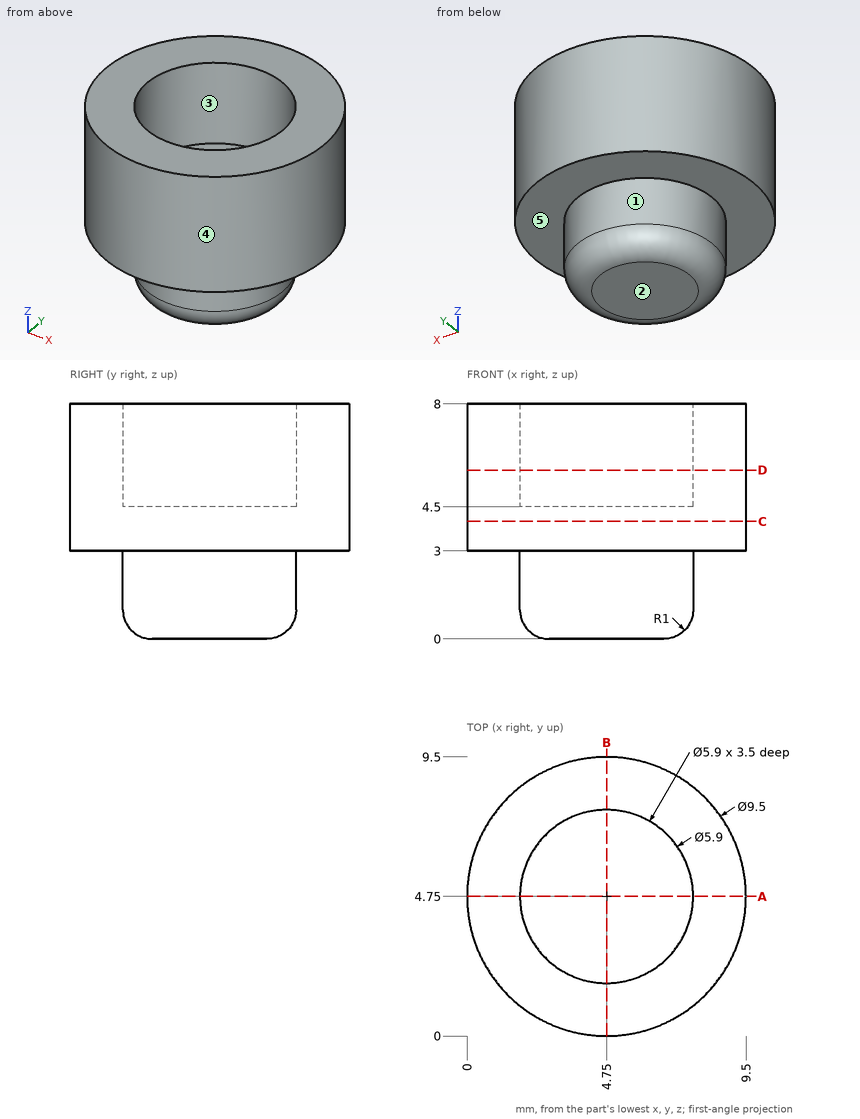
Geometry check sheet. Reference: drawing and pictorial views, mm from the part's lowest x, y, z. A direction names the side the tool comes from. Round coordinates to 2 decimals unless told otherwise and drop trailing zeros. Write each loop counter-clockwise with the first axis right and the second up, starting at its lowest first coordinate (ties: lowest second). Pieces come first, ordered by that corner, then holes. Notation, with made-up numbers: (23.5, -7) -> (57.5, -7) arc R24 ccw to (57.5, 21) -> close; hole circle Ø4 at (38.5, 10.25). An arc over 180 degrees is marked (long way). Put each result on its own line as item: value.
1) Access from +Z, -Z, +X, -X, +Y, -Y to the whole of each face (thin tool, end or side, straight path). Record for the marked faces 4 and 5.
Recorded:
face 4: +Z, -Z
face 5: -Z
2) Release check for a two-part mould opening along X. For the marked faces 1, 2 and 3 record: pulls with the +X half, pulls with the -X half, needs draft (parallel to the pull), parting line crosses it, or undercut.
Recorded:
face 1: parting line crosses it
face 2: needs draft
face 3: undercut
3) Cross-section at D-D, the plane z = 5.75. Enter the section's corners in (x, y).
Recorded:
outline: circle Ø9.5 at (4.75, 4.75); hole circle Ø5.9 at (4.75, 4.75)
4) Thickness scan on probe 1 along Y at (x, z) = (4.75, 7.3); probe 2 along Z at (x, y) = (8.5, 6); probe 3 along X at (y, z) = (7, 7.75). Record the ranges inside material, lowest first. Write a range as from..to.
Recorded:
probe 1: y = 0..1.8, 7.7..9.5
probe 2: z = 3..8
probe 3: x = 0.57..2.84, 6.66..8.93
5) Depth check by flat-ended pin: P1, Ø3, axis at x = 6, y = 5, coming from the +Z side; P2, Ø4, axis at x = 2, z = 3, coming from the +Y side; P3, Ø1, axis at y = 3.5, z = 1, coming from the +X side. Enter the tip coordinate at first touch or a pass-through.
Recorded:
P1: stops at z = 4.5
P2: stops at y = 9.44
P3: stops at x = 7.6
6) Cross-section at A-A, the plane y = 4.75. Enter the section's corners in (x, z).
Recorded:
outline: (0, 3) -> (1.8, 3) -> (1.8, 1) arc R1 ccw to (2.8, 0) -> (6.7, 0) arc R1 ccw to (7.7, 1) -> (7.7, 3) -> (9.5, 3) -> (9.5, 8) -> (7.7, 8) -> (7.7, 4.5) -> (1.8, 4.5) -> (1.8, 8) -> (0, 8) -> close
7) Cross-section at C-C, the plane z = 4. Enter the section's corners in (x, y).
Recorded:
outline: circle Ø9.5 at (4.75, 4.75)
